from build123d import *

# Parameters (mm, degrees)
F1_DEPTH      = 30
F2_W          = 18
F2_H          = 20
F2_H_2        = 50
F3_DEPTH      = 25
F2_H_3        = 90
F4_DEPTH      = 38
F6_DEPTH      = 8
F7_DEPTH      = 8
F9_DEPTH      = 10
F9_DEPTH_BACK = 34
F10_W         = 24
F10_H         = 17
F11_DEPTH     = 10.3313027798
F12_R         = 8
F13_DEPTH     = 52.001


with BuildPart() as f1:
    # F0 (on Right) → F1 (new body, symmetric)
    with BuildSketch(Plane.YZ):
        Polygon((-25, 58), (-45, 0), (45, 0), (25, 58), align=None)
    extrude(amount=F1_DEPTH, both=True)

    # F2 (on face) → F3 (cut)
    with BuildSketch(Plane.XY.offset(58)):
        with Locations((21, -35)):
            Rectangle(F2_W, F2_H)
        with Locations((21, 0)):
            Rectangle(F2_W, F2_H_2)
        with Locations((21, 35)):
            Rectangle(F2_W, F2_H)
    extrude(amount=-F3_DEPTH, mode=Mode.SUBTRACT)

    # F2 (on face) → F4 (cut)
    with BuildSketch(Plane.XY.offset(58)):
        with Locations((21, 0)):
            Rectangle(F2_W, F2_H_3)
        with Locations((-21, 0)):
            Rectangle(F2_W, F2_H_3)
    extrude(amount=-F4_DEPTH, mode=Mode.SUBTRACT)

    # F5 (on Right) → F6 (join, symmetric)
    with BuildSketch(Plane.YZ):
        Polygon((-29.4827586207, 45), (-41.5517241379, 45), (-41.5517241379, 10), align=None)
        Polygon((41.5517241379, 10), (41.5517241379, 45), (29.4827586207, 45), align=None)
    extrude(amount=F6_DEPTH, both=True)

    # F5 (on Right) → F7 (join, symmetric)
    with BuildSketch(Plane.YZ):
        Polygon((-29.4827586207, 45), (-41.5517241379, 45), (-41.5517241379, 10), align=None)
        Polygon((41.5517241379, 10), (41.5517241379, 45), (29.4827586207, 45), align=None)
    extrude(amount=F7_DEPTH, both=True)

    # F8 (on face) → F9 (join, two sides)
    with BuildSketch(Plane.YZ.offset(12)) as f9_sk:
        with BuildLine():
            ThreePointArc((-18.3303027798, 58), (-4.0861928738, 30.4218737414), (20, 50))
            ThreePointArc((20, 50), (19.5781262586, 54.0861928738), (18.3303027798, 58))
            Line((18.3303027798, 58), (-18.3303027798, 58))
        make_face()
        with BuildLine():
            Line((-18.3303027798, 58), (18.3303027798, 58))
            ThreePointArc((18.3303027798, 58), (0, 70), (-18.3303027798, 58))
        make_face()
    extrude(amount=F9_DEPTH)
    extrude(f9_sk.sketch, amount=-F9_DEPTH_BACK)

    # F10 (on face) → F11 (cut, through all)
    with BuildSketch(Plane.XY.offset(58)):
        with Locations((0, -16.5)):
            Rectangle(F10_W, F10_H)
        with Locations((0, 16.5)):
            Rectangle(F10_W, F10_H)
    extrude(amount=F11_DEPTH, mode=Mode.SUBTRACT)

    # F12 (on face) → F13 (cut, through all)
    with BuildSketch(Plane.YZ.offset(22)):
        with Locations((0, 50)):
            Circle(F12_R)
    extrude(amount=-F13_DEPTH, mode=Mode.SUBTRACT)


solid = f1.part
Read the model definition and answer for the solid it produces. Units are mm, in the model's axes. A direction names the side the tool comes from. Round coordinates to 2 decimals unless told otherwise and drop trailing zeros. Loops run counter-clockwise (first coordinate to the right, second up) from the corner with the lowest first, then second, coordinate; pieces in that order, holes last. Notation, with made-up numbers: (-5, 16.25) - (33, 16.25) arc R28 cw to (33, 42.25) - close; hole circle Ø10 at (63, -31). An arc over 180 degrees is marked (long way). One line per question, with ' | ' between items. Start each with the question number.
Q1. Section C-C on x = 0 is taken. Give the vertices of the cut face in (y, z).
Q2. Find the intervals of material crossed by L1, parallel to Z at x = -17, y = 0; L2, parallel to Z at x = -7, y = 0; L3, parallel to X at y = -40.5, z = 39.5, in increasing order.
Q3. Flat-ended cylindrical pins translate along their axes: pin 1 (3.5 mm diameter, centred on y = -33.5, z = 33.5, fed in from +X); pin 2 (13.5 mm diameter, centred on y = -35.5, z = 32.5, fed in from -X); pin 3 (9 mm diameter, centred on x = 24, y = 12, fed in from +Z); pin 4 (14.5 mm diameter, centred on y = 0, z = 50, fed in from +X). Find the tip coordinate at first contact, or state that the pin passes through.
Q4. Section A-A on x = -14 is taken. Give the vertices of the cut face in (y, z), plus the area to 3 significant figures.
Q5. Section D-D on y = -36 is taken. Give the vertices of the cut face in (x, z), plus the area to 3 significant figures.
Q6. For faces 1 (the flat face through (-8, 38, 36)), 2 (the flat face through (0, 17, 58)), 3 (the flat face through (0, -41.552, 28)), 4 (the flat face through (-8, -37, 32)), 5 (the flat face through (0, 41.552, 27)), determine the directions among +Z, -Z, +X, -X, +Y, -Y from which every point of the face is accessible in a straight line to the end or side of a thin tool.
Q7. Section B-B on y = 0 is taken. Give the vertices of the cut face in (x, z), plus the area to 3 significant figures.
Q8. For a pull along X with two mould halves and no side action, classify faces 6 (the flat face through (8, -37, 32)), 7 (the flat face through (-12, -1, 27)), 8 (the flat face through (-12, 12, 62)) as +X half, -X half, draft (parallel to the pull), parting line (faces both ways), or undercut.
Established:
1) outline: (-45, 0) - (45, 0) - (41.55, 10) - (41.55, 45) - (29.48, 45) - (25, 58) - (8, 58) - (8, 68.33) arc R20 ccw to (-8, 68.33) - (-8, 58) - (-25, 58) - (-29.48, 45) - (-41.55, 45) - (-41.55, 10) - close; hole circle Ø16 at (0, 50)
2) L1: 0 to 20, 30 to 42, 58 to 70 | L2: 0 to 42, 58 to 70 | L3: -8 to 8
3) pin 1: x = 12 | pin 2: x = -12 | pin 3: z = 68.34 | pin 4: through
4) outline: (-45, 0) - (45, 0) - (38.1, 20) - (-38.1, 20) - close; circle Ø40 at (0, 50); hole circle Ø16 at (0, 50) | area: 2,720 mm²
5) outline: (-30, 0) - (30, 0) - (30, 20) - (12, 20) - (12, 26.1) - (8, 26.1) - (8, 45) - (-8, 45) - (-8, 26.1) - (-12, 26.1) - (-12, 20) - (-30, 20) - close | area: 1,650 mm²
6) face 1: +Z, -X, +Y | face 2: +Z, +Y | face 3: +Z, +X, -X, -Y | face 4: +Z, -X, -Y | face 5: +Z, +X, -X, +Y
7) outline: (-30, 0) - (30, 0) - (30, 20) - (12, 20) - (12, 30) - (22, 30) - (22, 42) - (-22, 42) - (-22, 30) - (-12, 30) - (-12, 20) - (-30, 20) - close; (-22, 58) - (22, 58) - (22, 70) - (-22, 70) - close | area: 2,500 mm²
8) face 6: +X half | face 7: -X half | face 8: undercut
